Build history of the part. All positions in model axes, mm. Face numbers are marked on the shaded views. Coordinates: 2 decimals unless noted, no trailing zeros. Loops run counter-clockwise (first coordinate to the right, second up) from the corner with the lowest first, then second, coordinate; pieces in that order, holes last.
(1) Two-plate mould, pull along Y, no slides. Class the marked faces 1 and 2: pulls with the +Y half, pulls with the -Y half, needs draft (parallel to the pull), parting line crosses it, or undercut.
(2) Wall check: L1, parallel to X at y = 6, z = 9.5; L2, parallel to X at y = 7.5, z = 3.75; L3, parallel to X at y = -32.5, z = 4.25. Give the ranges that are in metal, low to high.
(3) Slice it at B-B (y = 19.5). Give the cut face in (x, z), and give its area (3 significant figures).
(4) Slice it at C-C (x = 7.5). Give the cut face in (y, z).
(5) Slice it at A-A (x = -13.5). Give the cut face in (y, z), and give its area (3 significant figures).
(6) Flat gauge pins, fed straight in: P1, Ø3.5, axis at x = 22.5, z = 5, coming from the +Y side; P2, Ø0.6, axis at x = -6, z = 3.5, coming from the +Y side; P3, Ø2, axis at x = -3.5, z = 3, coming from the +Y side. Where does each tip first touch, or does it go through?
from build123d import *

# Parameters (mm, degrees)
F0_R     = 37.4226300925
F1_DEPTH = 10


with BuildPart() as f1:
    # F0 (on Top) → F1 (new body)
    with BuildSketch(Plane.XY):
        Circle(F0_R)
        with BuildLine():
            ThreePointArc((-8.5269049855, 34.5365748806), (-5.4052755249, 35.1605760706), (-2.2403607921, 35.5030125009))
            ThreePointArc((-2.2403607921, 35.5030125009), (-0.0668734001, 35.5735666059), (2.1068638934, 35.5111846839))
            ThreePointArc((2.1068638934, 35.5111846839), (5.5820572148, 35.1329439468), (9.0033478551, 34.4154447962))
            Line((9.0033478551, 34.4154447962), (5.3277746774, 32.3108322918))
            Line((5.3277746774, 32.3108322918), (6.6450131126, 32.3108322918))
            Line((6.6450131126, 32.3108322918), (9.8926773092, 34.1704265231))
            ThreePointArc((9.8926773092, 34.1704265231), (18.0341344438, 30.6635468917), (25.0557426886, 25.2525814807))
            Line((25.0557426886, 25.2525814807), (20.8670180282, 25.2525814807))
            Line((20.8670180282, 25.2525814807), (21.6717198491, 24.5820395648))
            Line((21.6717198491, 24.5820395648), (25.7139348204, 24.5820395648))
            ThreePointArc((25.7139348204, 24.5820395648), (30.970985058, 17.5008913388), (34.3244938146, 9.3441017486))
            Line((34.3244938146, 9.3441017486), (30.6226182729, 11.4265037701))
            Line((30.6226182729, 11.4265037701), (30.9700332582, 10.5129266158))
            Line((30.9700332582, 10.5129266158), (34.5408713256, 8.5094841905))
            ThreePointArc((34.5408713256, 8.5094841905), (35.1576024678, 5.4245831021), (35.4993763194, 2.2972579413))
            ThreePointArc((35.4993763194, 2.2972579413), (33.326526558, -0.0646682307), (35.4901936241, -2.4350091671))
            ThreePointArc((35.4901936241, -2.4350091671), (35.1114069781, -5.7159612611), (34.4299693949, -8.9476432978))
            Line((34.4299693949, -8.9476432978), (32.3091186583, -5.346425809))
            Line((32.3091186583, -5.346425809), (32.1022830904, -6.364681758))
            Line((32.1022830904, -6.364681758), (34.1735842261, -9.8817637222))
            ThreePointArc((34.1735842261, -9.8817637222), (33.1529686946, -12.898208397), (31.8666911327, -15.8112968908))
            ThreePointArc((31.8666911327, -15.8112968908), (30.841049084, -17.7288692397), (29.700156108, -19.5801899959))
            ThreePointArc((29.700156108, -19.5801899959), (27.6349933602, -22.4006753268), (25.3029755485, -25.0048503597))
            Line((25.3029755485, -25.0048503597), (25.3181142434, -20.7694043622))
            Line((25.3181142434, -20.7694043622), (24.6594950259, -21.9101663099))
            Line((24.6594950259, -21.9101663099), (24.6461187726, -25.6525231228))
            ThreePointArc((24.6461187726, -25.6525231228), (17.5414682427, -30.9480210192), (9.3484371144, -34.3233133108))
            Line((9.3484371144, -34.3233133108), (11.4183174446, -30.5898860097))
            Line((11.4183174446, -30.5898860097), (10.4497633874, -31.0920979828))
            Line((10.4497633874, -31.0920979828), (8.4997417198, -34.543270022))
            ThreePointArc((8.4997417198, -34.543270022), (5.4306890655, -35.1566598156), (2.3196007667, -35.4979233956))
            ThreePointArc((2.3196007667, -35.4979233956), (0.0172965119, -33.3822489231), (-2.2828140972, -35.5003080679))
            ThreePointArc((-2.2828140972, -35.5003080679), (-5.7550130369, -35.1050272477), (-9.1716738253, -34.3709690343))
            Line((-9.1716738253, -34.3709690343), (-5.4097990505, -32.2477370501))
            Line((-5.4097990505, -32.2477370501), (-6.5905414522, -32.2477370501))
            Line((-6.5905414522, -32.2477370501), (-9.885855651, -34.1724007229))
            ThreePointArc((-9.885855651, -34.1724007229), (-18.0434280361, -30.6580791607), (-25.0760843465, -25.2323821104))
            Line((-25.0760843465, -25.2323821104), (-20.8179873924, -25.2323821104))
            Line((-20.8179873924, -25.2323821104), (-21.7606406659, -24.5914589614))
            Line((-21.7606406659, -24.5914589614), (-25.7049267509, -24.5914589614))
            ThreePointArc((-25.7049267509, -24.5914589614), (-27.7738883496, -22.2282306777), (-29.6263303406, -19.6917156101))
            ThreePointArc((-29.6263303406, -19.6917156101), (-30.7741756839, -17.8446973663), (-31.8070200014, -15.930994688))
            ThreePointArc((-31.8070200014, -15.930994688), (-33.2170505751, -12.73226862), (-34.3063234036, -9.4105944365))
            Line((-34.3063234036, -9.4105944365), (-30.6458889209, -11.5414279296))
            Line((-30.6458889209, -11.5414279296), (-31.3045081384, -10.400665982))
            Line((-31.3045081384, -10.400665982), (-34.5387960818, -8.5179034004))
            ThreePointArc((-34.5387960818, -8.5179034004), (-35.1643257366, -5.3808278739), (-35.505521273, -2.20024368))
            ThreePointArc((-35.505521273, -2.20024368), (-33.4584605706, 0.0814176869), (-35.4943927242, 2.3730145927))
            ThreePointArc((-35.4943927242, 2.3730145927), (-35.1180774116, 5.6748349785), (-34.435293299, 8.9271321558))
            Line((-34.435293299, 8.9271321558), (-32.2886370122, 5.4360465147))
            Line((-32.2886370122, 5.4360465147), (-31.8586565554, 6.4034969546))
            Line((-31.8586565554, 6.4034969546), (-34.1168341585, 10.0759485966))
            ThreePointArc((-34.1168341585, 10.0759485966), (-30.6126401352, 18.1204132699), (-25.2459538538, 25.0624206159))
            Line((-25.2459538538, 25.0624206159), (-25.2459538538, 20.6894481147))
            Line((-25.2459538538, 20.6894481147), (-24.5687514544, 21.6902010143))
            Line((-24.5687514544, 21.6902010143), (-24.5687514544, 25.7266314369))
            ThreePointArc((-24.5687514544, 25.7266314369), (-17.5076688048, 30.9671543113), (-9.3768544488, 34.3155608109))
            Line((-9.3768544488, 34.3155608109), (-11.3971997052, 30.6179970503))
            Line((-11.3971997052, 30.6179970503), (-10.4683693498, 30.9792086482))
            Line((-10.4683693498, 30.9792086482), (-8.5269049855, 34.5365748806))
        make_face(mode=Mode.SUBTRACT)
        with BuildLine():
            ThreePointArc((2.1068638934, 35.5111846839), (-0.0668734001, 35.5735666059), (-2.2403607921, 35.5030125009))
            ThreePointArc((-2.2403607921, 35.5030125009), (-0.0629027102, 33.4613425852), (2.1068638934, 35.5111846839))
        make_face()
    extrude(amount=F1_DEPTH)


solid = f1.part
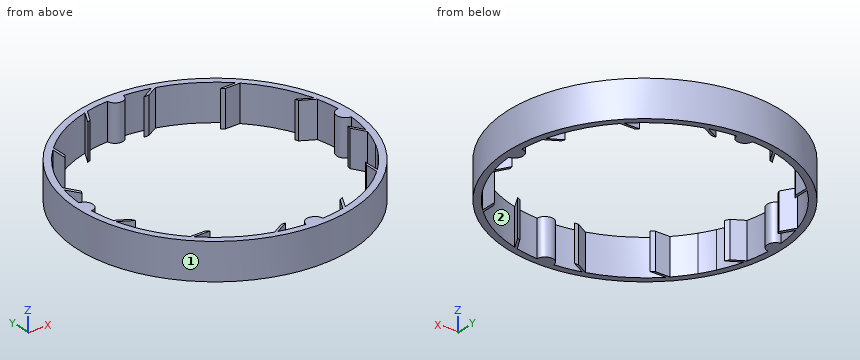
Response values:
1. face 1: parting line crosses it
1. face 2: undercut
2. L1: x = -36.94 to -35.06, -32.64 to -32.04, 35.06 to 36.94
2. L2: x = -36.66 to -34.77, -33.56 to -32.53, 34.77 to 36.66
2. L3: x = -18.55 to -14.46, -7.02 to -5.86, 9.65 to 10.36, 14.46 to 18.55
3. outline: (-31.94, 0) - (-29.75, 0) - (-29.75, 10) - (-31.94, 10) - close; (29.75, 0) - (31.94, 0) - (31.94, 10) - (29.75, 10) - close
3. area: 43.8 mm2
4. outline: (-36.66, 0) - (-34.77, 0) - (-34.77, 10) - (-36.66, 10) - close; (32.8, 0) - (33.55, 0) - (33.55, 10) - (32.8, 10) - close; (34.77, 0) - (36.66, 0) - (36.66, 10) - (34.77, 10) - close
5. outline: (-34.9, 0) - (-32.91, 0) - (-32.91, 10) - (-34.9, 10) - close; (32.91, 0) - (34.9, 0) - (34.9, 10) - (32.91, 10) - close
5. area: 39.8 mm2
6. P1: stops at y = 31.14
6. P2: stops at y = 36.99
6. P3: stops at y = 37.34
